Part model, mm, in its own coordinate system. Face numbers are marked on the shaded views. A direction names the side the tool comes from. Coordinates: 2 decimals unless noted, no trailing zeros. Loops run counter-clockwise (first coordinate to the right, second up) from the corner with the lowest first, then second, coordinate; pieces in that order, holes last. Notation, with made-up numbers: (-20, -7.5) - (29, -7.5) arc R9 ccw to (29, 4.5) - close; hole circle Ø7 at (-35.5, 55). An arc over 180 degrees is marked (long way). Answer as CSV lines item,"result".
Solid Edge part; units mm, degrees
sketch "Sketch1" plane through (0, 0, 0) normal (0, 0, 1) x (1, 0, 0)
  circle A0 centre (0, 0) radius 6.5
  circle A1 centre (0, 0) radius 3.75
extrude "Protrusion1" add sketch "Sketch1" along normal blind 5
sketch "Sketch2" plane through (0, 0, 0) normal (0, 0, 1) x (1, 0, 0)
  line L0 (0, 2.75) -> (8.1337, 2.75)
  line L1 (8.1337, 2.75) -> (8.1337, -2.75)
  line L2 (8.1337, -2.75) -> (0, -2.75)
  line L3 (0, -2.75) -> (0, 2.75)
extrude "Cutout1" cut sketch "Sketch2" along normal through all
fillet "Round_1" radius 1 2 edges at (5.8896, -2.75, 2.5) (5.8896, 2.75, 2.5)
sketch "Sketch3" plane through (0, 0, 0) normal (1, 0, 0) x (0, 1, 0)
  line L0 (4.25, 0) -> (9.3955, 1.3787)
revolve "RevolvedCutout1" cut sketch "Sketch3" angle 360 about axis through (0, 0, -57) along (0, 0, 1) material side at (0, 6.8357, 0.6411)
properties material "ABS Plastic, medium impact"
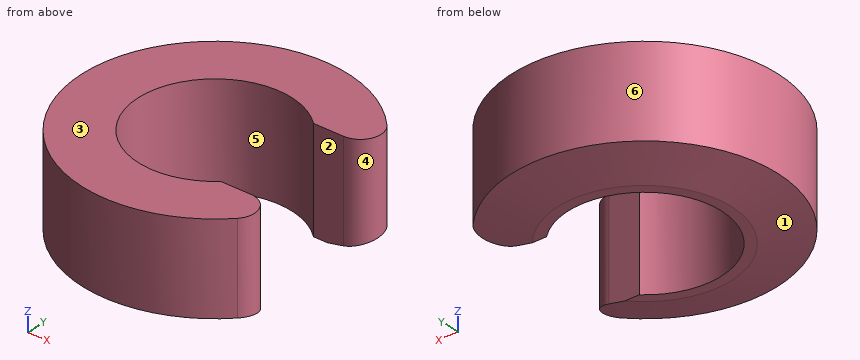
Q1. Flat gauge pins, fed straight in: pin 1 (1.5 mm diameter, centred on x = 3, z = 1, fed in from -Y); pin 2 (0.7 mm diameter, centred on x = 3, z = 3, fed in from +Y); pin 3 (1.5 mm diameter, centred on x = 3.5, y = -4.5, fed in from -Z). Where does each tip first touch, or does it go through?
Results:
pin 1,"stops at y = -6.1"
pin 2,"stops at y = 5.94"
pin 3,"stops at z = 0.19"
Q2. Wall check: L1, parallel to Y at x = 0, z = 3.3; L2, parallel to X at y = 0, z = 4; L3, parallel to Y at x = -2.25, z = 3. Give the ranges that are in metal, low to high.
Results:
L1,"y = -6.5 to -3.75, 3.75 to 6.5"
L2,"x = -6.5 to -3.75"
L3,"y = -6.1 to -3, 3 to 6.1"
Q3. Saw through at B-B (z = 3.25). Give the cut face in (x, y), then the cut area to 3 significant figures.
Results:
outline,"(2.55, -2.75) arc R3.75 cw (long way) to (2.55, 2.75) - (4.02, 2.75) arc R1 ccw to (4.75, 4.43) arc R6.5 ccw (long way) to (4.75, -4.43) arc R1 ccw to (4.02, -2.75) - close"
area,"70.7 mm^2"
Q4. Two-plate mould, pull along Y, no slides. Class the marked faces 3, 4, 5 and 6: released by +Y, released by -Y, zero draft, split by the parting line, or undercut.
Results:
face 3,"zero draft"
face 4,"undercut"
face 5,"undercut"
face 6,"split by the parting line"
Q5. Saw through at A-A (x = 0). Give the cut face in (y, z).
Results:
outline,"(-6.5, 0.6) - (-4.25, 0) - (-3.75, 0) - (-3.75, 5) - (-6.5, 5) - close; (3.75, 0) - (4.25, 0) - (6.5, 0.6) - (6.5, 5) - (3.75, 5) - close"
Q6. Which spindle directions (+Z, -Z, +X, -X, +Y, -Y) get a long thin tool onto all of the face, cutting with end or side? Do the marked faces 1 and 2. Say none if no direction does.
Results:
face 1,"-Z"
face 2,"+Z, -Z, +X"
Q7. Saw through at C-C (y = 0). Give the cut face in (x, z).
Results:
outline,"(-6.5, 0.6) - (-4.25, 0) - (-3.75, 0) - (-3.75, 5) - (-6.5, 5) - close"
